from build123d import *

# Parameters (mm, degrees)
F0_W     = 76.2
F0_H     = 3.4163
F1_DEPTH = 3.4163


with BuildPart() as f1:
    # F0 (on Right) → F1 (new body)
    with BuildSketch(Plane.YZ):
        Polygon((-50.8, 0), (-50.8, -6.35), (50.8, -6.35), (50.8, 0), (110.8837, 0), (110.8837, 133.35), (114.3, 133.35), (114.3, 234.95), (110.8837, 234.95), (110.8837, 374.65), (114.3, 374.65), (114.3, 476.25), (110.8837, 476.25), (110.8837, 615.95), (114.3, 615.95), (114.3, 717.55), (110.8837, 717.55), (110.8837, 857.25), (38.1, 857.25), (-38.1, 857.25), (-110.8837, 857.25), (-110.8837, 717.55), (-114.3, 717.55), (-114.3, 615.95), (-110.8837, 615.95), (-110.8837, 476.25), (-114.3, 476.25), (-114.3, 374.65), (-110.8837, 374.65), (-110.8837, 234.95), (-114.3, 234.95), (-114.3, 133.35), (-110.8837, 133.35), (-110.8837, 0), align=None)
        with Locations((0, 846.01685)):
            Rectangle(F0_W, F0_H, mode=Mode.SUBTRACT)
    extrude(amount=F1_DEPTH)


solid = f1.part
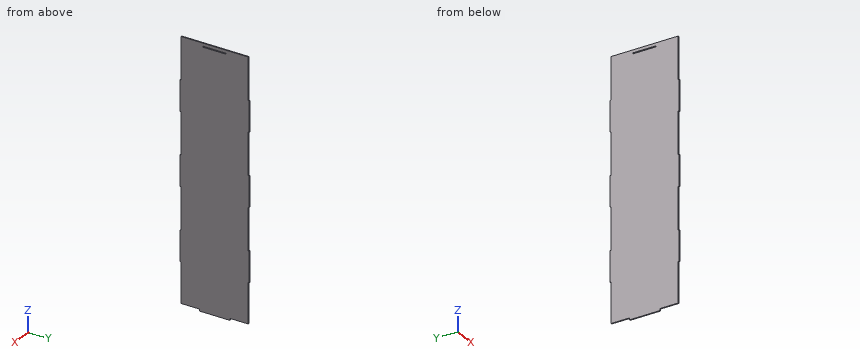
Design review of the part built by this model. Coordinates are the model's own, in mm. Give positions to 0.01 mm unless a question says otherwise; leave off trailing zeros. Loops run counter-clockwise (first coordinate to the right, second up) from the corner with the lowest first, then second, coordinate; pieces in that order, holes last. Notation, with made-up numbers: (69, 34.5) - (99, 34.5) arc R17 ccw to (99, 63.5) - close; hole circle Ø8 at (59, 27). An arc over 180 degrees is marked (long way). Write item = value, one per line.
1) To check wall thickness, follow line 1 (Z direction, x = 2.4, y = -9.5) (3 decimals); line 2 (Z direction, x = 1.3, y = -91); line 3 (Y direction, x = 2.7, z = 533.5). State the ranges of each line that lie inside material, in increasing order.
Result sheet:
line_1 = -6.35 to 844.309, 847.725 to 857.25
line_2 = 0 to 857.25
line_3 = -110.88 to 110.88
2) Take a section at A-A on z = 287.5. State the section outline as (x, y) points, and give its area (3 significant figures).
Result sheet:
outline = (0, -110.88) - (3.42, -110.88) - (3.42, 110.88) - (0, 110.88) - close
area = 758 mm2
3) Clearance check with flat-ended pins moving along their axes: pin 1 Ø1 at (x, y) = (2, -113) entering from -Z; pin 2 Ø1 at (x, y) = (1, -69) entering from -Z; pin 3 Ø1.7 at (x, y) = (1, -112.5) entering from +Z. State where each tip first meets the part, or that it passes through.
Result sheet:
pin_1 = 133.35
pin_2 = 0
pin_3 = 717.55
